Input: part model. Units: mm. Frame: model coordinates. Coordinates: 2 decimals unless noted, no trailing zeros. Order: outer loops, then holes, each group sorted by start corner. A loop starts at its lowest first (then second) coordinate and runs counter-clockwise, first axis right, second up. Notation, with made-up numbers: (61.5, 86) -> (106.5, 86) arc R18 ccw to (106.5, 101) -> close; hole circle Ø3 at (-12.75, 20.5). An arc over 180 degrees is marked (long way). One line per question, with ' | ' between items.
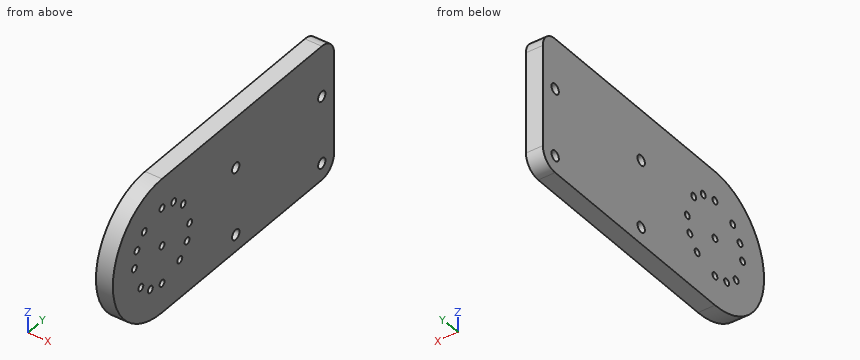
Autodesk Inventor part; units mm, degrees
ref_plane "YZ Plane" through (0, 0, 0) normal (1, 0, 0) x (0, 1, 0)
ref_plane "XZ Plane" through (0, 0, 0) normal (0, 1, 0) x (-1, 0, 0)
ref_plane "XY Plane" through (0, 0, 0) normal (0, 0, 1) x (1, 0, 0)
sketch "Sketch2" plane through (0, 0, 0) normal (1, 0, 0) x (0, 1, 0)
  circle A0 centre (0, 0) radius 11.25
  circle A1 centre (11.25, 0) radius 1
  circle A2 centre (0, 11.25) radius 1
  circle A3 centre (-11.25, 0) radius 1
  circle A4 centre (0, -11.25) radius 1
  circle A5 centre (7.2314, -8.618) radius 1
  line L0 (0, 0) -> (7.2314, -8.618)
  line L1 (0, 0) -> (11.25, 0)
  circle A6 centre (8.618, 7.2314) radius 1
  circle A7 centre (-7.2314, 8.618) radius 1
  circle A8 centre (-8.618, -7.2314) radius 1
  circle A9 centre (10.196, -4.7545) radius 1
  line L2 (0, 0) -> (10.196, -4.7545)
  circle A10 centre (4.7545, 10.196) radius 1
  circle A11 centre (-10.196, 4.7545) radius 1
  circle A12 centre (-4.7545, -10.196) radius 1
  circle A13 centre (0, 0) radius 20
  line L3 (0, 20) -> (70, 20)
  line L4 (70, 20) -> (70, -20)
  line L5 (70, -20) -> (0, -20)
  line L6 (0, -20) -> (0, 20)
  line L7 (70, 20) -> (0, 20)
  line L8 (0, 20) -> (0, 15)
  line L9 (0, 15) -> (70, 15)
  line L10 (70, 15) -> (70, 20)
  circle A14 centre (0, 0) radius 1
  point P0 (13.2288, 15)
  dimension "d0" = 22.5
  dimension "d1" = 2
  dimension "d4" = 360
  dimension "d6" = 2
  dimension "d7" = 50
  dimension "d10" = 360
  dimension "d12" = 2
  dimension "d13" = 25
  dimension "d16" = 360
  dimension "d18" = 40
  dimension "d19" = 70
  dimension "d20" = 5
  dimension "d21" = 2
extrude "Extrusion1" add sketch "Sketch2" along normal blind 5 contours A1 L1 A14 L6 A2 A0 A10 A6 | A0 A6 A10 A2 L6 L9 A13 A4 A5 A9 A1 | A0 A9 L2 A14 L1 A1 | A9 A0 A5 L0 A14 L2 | A14 L6 A4 A0 A12 A8 A3 A11 A7 A2 | L0 A5 A0 A4 L6 A14 | A0 A7 A11 A3 A8 A12 A4 L6 A13 A2 | L6 A13 L9 | A13 L9 L4 L5 | L3 L4 L9 A13
sketch "Sketch3" plane through (5, 0, 0) normal (1, 0, 0) x (0, 0, -1)
  circle A0 centre (-5, 65) radius 1.5
  line L0 (20, 70) -> (-20, 70)
  line L1 (-20, 70) -> (-20, 0)
  circle A1 centre (15, 65) radius 1.5
  circle A2 centre (-5, 30) radius 1.5
  circle A3 centre (15, 30) radius 1.5
  point P0 (0, 0)
  dimension "d24" = 5
  dimension "d25" = 15
  dimension "d26" = 3
  dimension "d29" = 20
  dimension "d32" = 35
extrude "Extrusion2" cut sketch "Sketch3" against normal blind 5
fillet "Fillet1" radius 5 2 edges at (2.5, 70, 20) (2.5, 70, -20)
properties part number "StereoVisionHolder_2"
1. Cut plane B-B, the plane x = 0.75. State how many separate pieces and enclosed holes the cut face has, and give its area (3 significant figures).
Recorded:
separate pieces: 1 | enclosed holes: 17 | area: 3,350 mm^2
2. Cut plane C-C, the plane z = 13.5. Return loops of the section in (x, y), and give its area (3 significant figures).
Recorded:
outline: (0, -14.76) -> (5, -14.76) -> (5, 70) -> (0, 70) -> close | area: 424 mm^2
3. Cut plane A-A, the plane z = 0. Return loops of the section in (x, y).
Recorded:
outline: (0, -20) -> (5, -20) -> (5, -12.25) -> (0, -12.25) -> close; (0, -10.25) -> (5, -10.25) -> (5, -1) -> (0, -1) -> close; (0, 1) -> (5, 1) -> (5, 10.25) -> (0, 10.25) -> close; (0, 12.25) -> (5, 12.25) -> (5, 70) -> (0, 70) -> close
4. Ray query, line 1 (Y direction, x = 2.45, z = 0); line 2 (Z direction, x = 1.5, y = 0); line 3 (Z direction, x = 4.45, y = -11). Return the intervals inside material, ascending. Write a range as [from, to].
Recorded:
line 1: y = [-20, -12.25], [-10.25, -1], [1, 10.25], [12.25, 70] | line 2: z = [-20, -12.25], [-10.25, -1], [1, 10.25], [12.25, 20] | line 3: z = [-16.7, -0.97], [0.97, 4.16], [5.35, 16.7]
5. Pin query (flat end, axial travel): pin 1 Ø1.8 at (y, z) = (65, 5) entering from -X. Return the tip coordinate at first contact, or that it passes through.
Recorded:
pin 1: passes through
